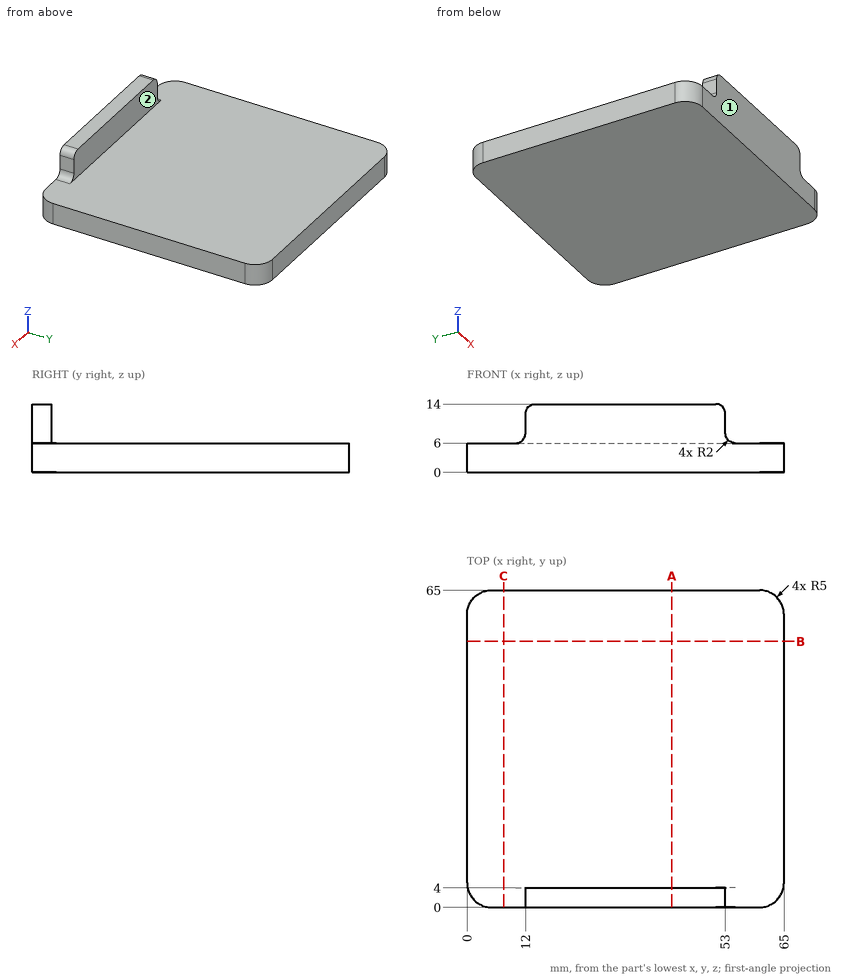
Verification items for this drawing (mm, ordinates from the low corner). A direction names the side the tool comes from. Coordinates: 2 decimals unless noted, no trailing zeros. Order: outer loops, then holes, each group sorted by start corner. A loop starts at its lowest first (then second) coordinate and runs counter-clockwise, first axis right, second up. Notation, with made-up numbers: M 8.5,30.25 L 44.5,30.25 A15 ccw 44.5,45.25 Z; hole C 12,25 d4. An arc over 180 degrees is marked long. One line per item, written item: value. Start each with the question number.
Item 1: Depth check by flat-ended pin: P1, Ø4.5, axis at y = 3, z = 9, coming from the +X side; P2, Ø2, axis at y = 2, z = 9.5, coming from the -X side; P3, Ø4, axis at x = 46, y = 37, coming from the +Z side. Enter the tip coordinate at first touch or a pass-through.
Item 2: Access from +Z, -Z, +X, -X, +Y, -Y to the whole of each face (thin tool, end or side, straight path). Record for the marked faces 1 and 2.
Item 3: Sectioned sample at B-B on y = 54.5. Record the cut outline in (x, z), then the cut area to 3 significant figures.
Item 4: Thickness scan on probe 1 along Y at (x, z) = (15, 9); probe 2 along Z at (x, y) = (30.5, 39.5); probe 3 along X at (y, z) = (4.5, 2). Record the ranges inside material, lowest first.
Item 5: Sectioned sample at A-A on x = 42. Record the cut outline in (y, z).
Calculated:
1. P1: x = 53.44
1. P2: x = 12
1. P3: z = 6
2. face 1: +Z, -Z, +X, -X, -Y
2. face 2: +Z, +X, -X, +Y
3. outline: M 0,0 L 65,0 L 65,6 L 0,6 Z
3. area: 390 mm^2
4. probe 1: 0 to 4
4. probe 2: 0 to 6
4. probe 3: 0.03 to 64.97
5. outline: M 0,0 L 65,0 L 65,6 L 4,6 L 4,14 L 0,14 Z
